Can you work these out from the model? Positions are in its coordinate system, mm. A direction names the side the tool comes from. Give positions to 0.01 mm unless a question says otherwise; leave off trailing zeros. Write each loop counter-clockwise with the first axis right and the second up, starting at its lowest first coordinate (ties: lowest second). Pieces come first, ordered by that corner, then holes.
1. Suppose I cut it at D-D (z = 103). Please give me the cut outline in (x, y), and give its area (3 significant figures).
2. On a 3-axis mill with a long thin cutter (end or side, diameter ignored), from which of +Z, -Z, +X, -X, +Y, -Y can I reach the whole of each face in a straight line? I mean faces 1 (the cylindrical face through (-91.273, -504.93, 119.035)), 2 (the flat face through (-65, -500, 2)). Say none if no direction works.
3. Suppose I cut it at B-B (y = -193.5). Please give me the cut outline in (x, z), and give its area (3 significant figures).
4. I'm going to push flat-ended pins straight in: pin 1 (13 mm diameter, centred on x = 64.95, z = -37.5, fed in from +Y); pin 2 (12 mm diameter, centred on y = -114.5, z = -15, fed in from +X); pin 3 (1.5 mm diameter, centred on x = 40.5, y = -350, fed in from +Z); pin 4 (10 mm diameter, centred on x = -59.5, y = -77.5, fed in from -Z). Where does each tip first touch, or does it pass through?
5. Suppose I cut it at C-C (x = 30.5). Please give me the cut outline in (y, z).
6. Thinking about a two-plate mould opening in Y: for faces 3 (the flat face through (2, -510, 2)), 4 (the flat face through (-39, 0, 39)), 5 (the cylindrical face through (15.02, -246.5, -47.69)), 6 (the cylindrical face through (-34.471, 4.93, 83.137)), which applies, pulls with the +Y half, pulls with the -Y half, needs draft (parallel to the pull), parting line crosses it, or undercut?
7. If I drill on probe 1 along Y at (x, z) = (32, -76); probe 2 along X at (y, z) = (6.5, 37.5); probe 3 along Y at (x, z) = (-39.5, -123.5), over which ranges is the centre line in solid material (lowest first)?
8. Suppose I cut it at A-A (z = 13.5). Please give me the cut outline in (x, y), and give its area (3 significant figures).
```python
from build123d import *

# Parameters (mm, degrees)
SKETCH_1_R      = 90
SKETCH_1_R_2    = 4.1
EXTRUDE_1_DEPTH = 10
SKETCH_2_R      = 50
EXTRUDE_2_DEPTH = 500
SKETCH_3_R      = 150
EXTRUDE_3_DEPTH = 10


with BuildPart() as part:
    # 草图1 → 凸台-拉伸1 (new body)
    with BuildSketch(Plane(origin=(0, 0, 0), x_dir=(1, 0, 0), z_dir=(0, 1, 0))):
        with Locations(Location((0, 0, 0), (0, 0, 270))):
            Circle(SKETCH_1_R)
        with Locations(Location((0, -75, 0), (0, 0, 270))):
            Circle(SKETCH_1_R_2, mode=Mode.SUBTRACT)
        with Locations(Location((-64.951905284, -37.5, 0), (0, 0, 270))):
            Circle(SKETCH_1_R_2, mode=Mode.SUBTRACT)
        with Locations(Location((-64.951905284, 37.5, 0), (0, 0, 270))):
            Circle(SKETCH_1_R_2, mode=Mode.SUBTRACT)
        with Locations(Location((0, 75, 0), (0, 0, 270))):
            Circle(SKETCH_1_R_2, mode=Mode.SUBTRACT)
        with Locations(Location((64.951905284, 37.5, 0), (0, 0, 270))):
            Circle(SKETCH_1_R_2, mode=Mode.SUBTRACT)
        with Locations(Location((64.951905284, -37.5, 0), (0, 0, 270))):
            Circle(SKETCH_1_R_2, mode=Mode.SUBTRACT)
    extrude(amount=EXTRUDE_1_DEPTH)

    # 草图2 → 凸台-拉伸2 (add)
    with BuildSketch(Plane.XZ):
        with Locations(Location((0, 0, 0), (0, 0, 270))):
            Circle(SKETCH_2_R)
    extrude(amount=EXTRUDE_2_DEPTH)

    # 草图3 → 凸台-拉伸3 (add)
    with BuildSketch(Plane.XZ.offset(500)):
        with Locations(Location((0, 0, 0), (0, 0, 270))):
            Circle(SKETCH_3_R)
    extrude(amount=EXTRUDE_3_DEPTH)


solid = part.part
```
Checks:
1. outline: (-109.05, -510) - (109.05, -510) - (109.05, -500) - (-109.05, -500) - close
1. area: 2,180 mm2
2. face 1: +Y, -Y
2. face 2: none
3. outline: circle Ø100 at (0, 0)
3. area: 7,850 mm2
4. pin 1: stops at y = 10
4. pin 2: stops at x = 49.18
4. pin 3: stops at z = 30.33
4. pin 4: passes through
5. outline: (-510, -146.87) - (-500, -146.87) - (-500, -39.62) - (0, -39.62) - (0, -84.67) - (10, -84.67) - (10, 84.67) - (0, 84.67) - (0, 39.62) - (-500, 39.62) - (-500, 146.87) - (-510, 146.87) - close
6. face 3: pulls with the -Y half
6. face 4: undercut
6. face 5: undercut
6. face 6: needs draft
7. probe 1: y = -510 to -500, 0 to 10
7. probe 2: x = -81.82 to -69.05, -60.85 to 60.85, 69.05 to 81.82
7. probe 3: y = -510 to -500
8. outline: (-149.39, -510) - (149.39, -510) - (149.39, -500) - (48.14, -500) - (48.14, 0) - (88.98, 0) - (88.98, 10) - (-88.98, 10) - (-88.98, 0) - (-48.14, 0) - (-48.14, -500) - (-149.39, -500) - close
8. area: 52,900 mm2
